Autodesk Inventor part; units mm, degrees
ref_plane "YZ Plane" through (0, 0, 0) normal (1, 0, 0) x (0, 1, 0)
ref_plane "XZ Plane" through (0, 0, 0) normal (0, 1, 0) x (-1, 0, 0)
ref_plane "XY Plane" through (0, 0, 0) normal (0, 0, 1) x (1, 0, 0)
sketch "Sketch1" plane through (0, 0, 0) normal (1, 0, 0) x (0, 1, 0)
  point P0 (0, 0)
sketch "Sketch2" plane through (0, 0, 0) normal (0, 1, 0) x (-1, 0, 0)
  line L0 (0, 0) -> (91.44, 0)
  line L1 (91.44, 0) -> (91.44, -457.2)
  line L2 (91.44, -457.2) -> (0, -457.2)
  line L3 (0, -457.2) -> (0, 0)
  dimension "d0" = 91.44
  dimension "d1" = 457.2
extrude "Extrusion1" add sketch "Sketch2" along normal blind 457.2
fillet "Fillet1" radius 60.96 2 edges at (-45.72, 457.2, 0) (-45.72, 457.2, -457.2)
sketch "Sketch3" plane through (0, 0, 0) normal (1, 0, 0) x (0, 0, -1)
  line L0 (150.961, 395.9055) -> (268.4404, 395.9055)
  line L1 (268.4404, 395.9055) -> (268.4404, 300.7472)
  line L2 (268.4404, 300.7472) -> (150.961, 300.7472)
  line L3 (150.961, 300.7472) -> (150.961, 395.9055)
  point P0 (0, 0)
extrude "Extrusion2" add sketch "Sketch3" along normal blind 25.4
properties part number "new tal lpart"
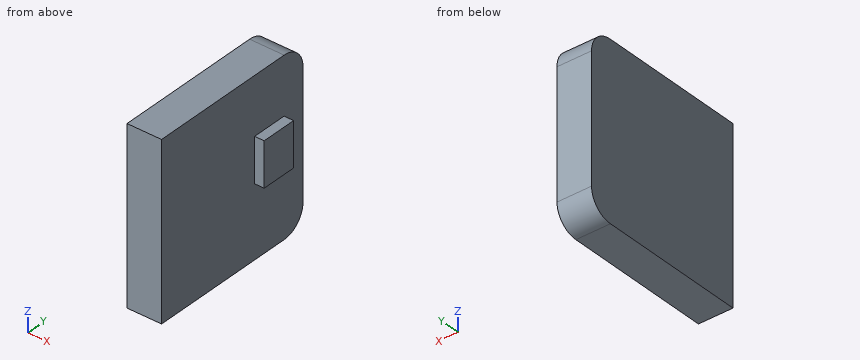
Read the model definition and answer for the solid it produces. Units are mm, in the model's axes. Round coordinates to 2 decimals unless told otherwise and drop trailing zeros. Write each loop counter-clockwise with the first axis right and the second up, starting at its lowest first coordinate (ties: lowest second). Pieces come first, ordered by that corner, then holes. Notation, with made-up numbers: (42, -29.75) - (93, -29.75) arc R37 ccw to (93, 8.25) - close; hole circle Ø11 at (-10, 12.5). An arc over 180 degrees is marked (long way). Use a Markdown table: item, result.
(1) The part is cut by section A-A (z = -159). Write down the section's boundary in (x, y).
Reported:
| item | result |
|---|---|
| outline | (-91.44, 0) - (0, 0) - (0, 300.75) - (25.4, 300.75) - (25.4, 395.91) - (0, 395.91) - (0, 457.2) - (-91.44, 457.2) - close |
(2) Each of these flat-tipped pins is pushed along its axis until it touches: pin 1 Ø2 at (y, z) = (238, -154) entering from +X; pin 2 Ø20.5 at (x, z) = (19, -197.5) entering from -Y; pin 3 Ø5 at (x, y) = (-48, 399) entering from +Z. Where does it stop, or does it pass through?
Reported:
| item | result |
|---|---|
| pin 1 | x = 0 |
| pin 2 | y = 300.75 |
| pin 3 | z = 0 |
(3) The part is cut by section D-D (z = -343). Write down the section's boundary in (x, y), then the cut area to 3 significant figures.
Reported:
| item | result |
|---|---|
| outline | (-91.44, 0) - (0, 0) - (0, 457.2) - (-91.44, 457.2) - close |
| area | 41,800 mm2 |
(4) The part is cut by section B-B (y = 337.5). Write down the section's boundary in (x, z).
Reported:
| item | result |
|---|---|
| outline | (-91.44, -457.2) - (0, -457.2) - (0, -268.44) - (25.4, -268.44) - (25.4, -150.96) - (0, -150.96) - (0, 0) - (-91.44, 0) - close |
(5) Straight lines are drawn through the part: line 1 along X through (y, z) = (410, -51.5); line 2 along Y through (x, z) = (15.5, -201); line 3 along Y through (x, z) = (-6.5, -397.5). For each, find the intervals that lie inside material, in ascending order. Write a range as [from, to].
Reported:
| item | result |
|---|---|
| line 1 | [-91.44, 0] |
| line 2 | [300.75, 395.91] |
| line 3 | [0, 457.19] |
(6) The part is cut by section C-C (y = 161). Write down the section's boundary in (x, z), then the cut area to 3 significant figures.
Reported:
| item | result |
|---|---|
| outline | (-91.44, -457.2) - (0, -457.2) - (0, 0) - (-91.44, 0) - close |
| area | 41,800 mm2 |
